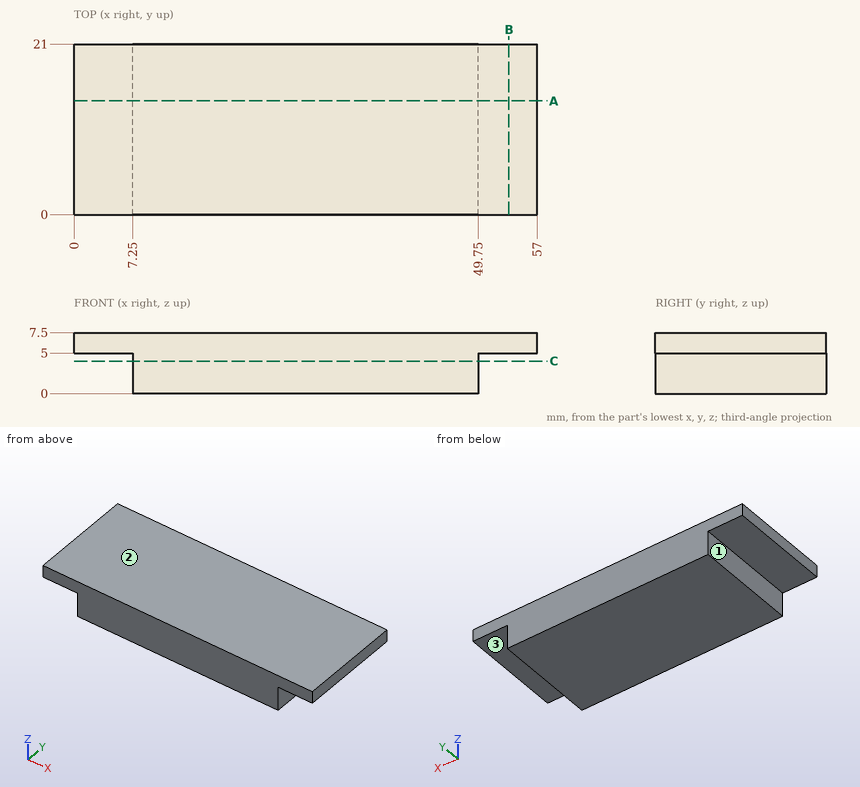
Geometry check sheet. Reference: drawing and pictorial views, mm from the part's lowest x, y, z. A direction names the side the tool comes from. Coordinates: 2 decimals unless noted, no trailing zeros. Write each loop counter-clockwise with the first axis right and the second up, starting at its lowest first coordinate (ties: lowest second). Pieces come first, ordered by that corner, then holes. Notation, with made-up numbers: (3, 62.25) - (21, 62.25) arc R13 ccw to (21, 67.25) - close; hole circle Ø11 at (52, 14.25). An arc over 180 degrees is marked (long way). Write item = value, one per line.
Q1. Material ranges on L1, parallel to X at y = 12.5, z = 0.5; L2, parallel to Z at x = 54, y = 2, recorded low to high. Write a range as from..to.
Answer:
L1 = 7.25..49.75
L2 = 5..7.5
Q2. Cross-section at C-C (z = 4). Enter the section's corners in (x, y).
Answer:
outline = (7.25, 0) - (49.75, 0) - (49.75, 21) - (7.25, 21) - close
Q3. Cross-section at A-A (y = 14). Enter the section's corners in (x, z).
Answer:
outline = (0, 5) - (7.25, 5) - (7.25, 0) - (49.75, 0) - (49.75, 5) - (57, 5) - (57, 7.5) - (0, 7.5) - close
Q4. Access from +Z, -Z, +X, -X, +Y, -Y to the whole of each face (thin tool, end or side, straight path). Record for the marked faces 1, 2 and 3.
Answer:
face_1 = -Z, -X, +Y, -Y
face_2 = +Z, +X, -X, +Y, -Y
face_3 = -Z, +X, +Y, -Y
Q5. Cross-section at B-B (x = 53.5). Enter the section's corners in (y, z), plus the area to 3 significant figures.
Answer:
outline = (0, 5) - (21, 5) - (21, 7.5) - (0, 7.5) - close
area = 52.5 mm²
Q6. Go/stop test with flat-tipped pins: pin 1 Ø4 at (y, z) = (7, 2.5) entering from +X; pin 2 Ø3.5 at (x, y) = (54.5, 8) entering from -Z; pin 3 Ø2.5 at (y, z) = (15.5, 1.5) entering from -X. Record where each tip stops, or that it passes through.
Answer:
pin_1 = 49.75
pin_2 = 5
pin_3 = 7.25
